```python
from build123d import *

# Parameters (mm, degrees)
F0_R     = 2.1463
F1_DEPTH = 380


with BuildPart() as f1:
    # F0 (on Front) → F1 (new body)
    with BuildSketch(Plane.XZ):
        with BuildLine():
            Line((-9.75241, 4.759444), (-12.019248, 4.759444))
            ThreePointArc((-12.019248, 4.759444), (-13.166227, 4.987592), (-14.138589, 5.637303))
            Line((-14.138589, 5.637303), (-16.393426, 7.892141))
            ThreePointArc((-16.393426, 7.892141), (-16.575125, 8.805603), (-15.800729, 9.323038))
            Line((-15.800729, 9.323038), (-13.692529, 9.323038))
            ThreePointArc((-13.692529, 9.323038), (-13.477003, 9.412312), (-13.387729, 9.627838))
            Line((-13.387729, 9.627838), (-13.387729, 10.339038))
            ThreePointArc((-13.387729, 10.339038), (-13.618353, 10.895814), (-14.175129, 11.126438))
            Line((-14.175129, 11.126438), (-18.874129, 11.126438))
            ThreePointArc((-18.874129, 11.126438), (-20.29301, 10.538718), (-20.880729, 9.119838))
            Line((-20.880729, 9.119838), (-20.880729, 4.420838))
            ThreePointArc((-20.880729, 4.420838), (-20.650105, 3.864062), (-20.093329, 3.633438))
            Line((-20.093329, 3.633438), (-19.382129, 3.633438))
            ThreePointArc((-19.382129, 3.633438), (-19.166603, 3.722712), (-19.077329, 3.938238))
            Line((-19.077329, 3.938238), (-19.077329, 6.046438))
            ThreePointArc((-19.077329, 6.046438), (-18.559895, 6.820834), (-17.646432, 6.639135))
            Line((-17.646432, 6.639135), (-15.391595, 4.384297))
            ThreePointArc((-15.391595, 4.384297), (-14.741884, 3.411936), (-14.513736, 2.264957))
            Line((-14.513736, 2.264957), (-14.513736, -0.001881))
            ThreePointArc((-14.513736, -0.001881), (-14.741884, -1.14886), (-15.391595, -2.121222))
            Line((-15.391595, -2.121222), (-17.646432, -4.376059))
            ThreePointArc((-17.646432, -4.376059), (-18.559895, -4.557758), (-19.077329, -3.783362))
            Line((-19.077329, -3.783362), (-19.077329, -1.675162))
            ThreePointArc((-19.077329, -1.675162), (-19.166603, -1.459636), (-19.382129, -1.370362))
            Line((-19.382129, -1.370362), (-20.093329, -1.370362))
            ThreePointArc((-20.093329, -1.370362), (-20.650105, -1.600986), (-20.880729, -2.157762))
            Line((-20.880729, -2.157762), (-20.880729, -6.856762))
            ThreePointArc((-20.880729, -6.856762), (-20.29301, -8.275643), (-18.874129, -8.863362))
            Line((-18.874129, -8.863362), (-14.175129, -8.863362))
            ThreePointArc((-14.175129, -8.863362), (-13.618353, -8.632738), (-13.387729, -8.075962))
            Line((-13.387729, -8.075962), (-13.387729, -7.364762))
            ThreePointArc((-13.387729, -7.364762), (-13.477003, -7.149236), (-13.692529, -7.059962))
            Line((-13.692529, -7.059962), (-15.800729, -7.059962))
            ThreePointArc((-15.800729, -7.059962), (-16.575125, -6.542528), (-16.393426, -5.629065))
            Line((-16.393426, -5.629065), (-14.138589, -3.374228))
            ThreePointArc((-14.138589, -3.374228), (-13.166227, -2.724517), (-12.019248, -2.496368))
            Line((-12.019248, -2.496368), (-9.75241, -2.496368))
            ThreePointArc((-9.75241, -2.496368), (-8.605431, -2.724517), (-7.63307, -3.374228))
            Line((-7.63307, -3.374228), (-5.378232, -5.629065))
            ThreePointArc((-5.378232, -5.629065), (-5.196534, -6.542528), (-5.970929, -7.059962))
            Line((-5.970929, -7.059962), (-8.079129, -7.059962))
            ThreePointArc((-8.079129, -7.059962), (-8.294656, -7.149236), (-8.383929, -7.364762))
            Line((-8.383929, -7.364762), (-8.383929, -8.075962))
            ThreePointArc((-8.383929, -8.075962), (-8.153305, -8.632738), (-7.596529, -8.863362))
            Line((-7.596529, -8.863362), (5.814671, -8.863362))
            ThreePointArc((5.814671, -8.863362), (6.371447, -8.632738), (6.602071, -8.075962))
            Line((6.602071, -8.075962), (6.602071, -7.364762))
            ThreePointArc((6.602071, -7.364762), (6.512797, -7.149236), (6.297271, -7.059962))
            Line((6.297271, -7.059962), (4.189071, -7.059962))
            ThreePointArc((4.189071, -7.059962), (3.414675, -6.542528), (3.596374, -5.629065))
            Line((3.596374, -5.629065), (5.851211, -3.374228))
            ThreePointArc((5.851211, -3.374228), (6.823573, -2.724517), (7.970552, -2.496368))
            Line((7.970552, -2.496368), (10.23739, -2.496368))
            ThreePointArc((10.23739, -2.496368), (11.384369, -2.724517), (12.35673, -3.374228))
            Line((12.35673, -3.374228), (14.611568, -5.629065))
            ThreePointArc((14.611568, -5.629065), (14.793266, -6.542528), (14.018871, -7.059962))
            Line((14.018871, -7.059962), (11.910671, -7.059962))
            ThreePointArc((11.910671, -7.059962), (11.695144, -7.149236), (11.605871, -7.364762))
            Line((11.605871, -7.364762), (11.605871, -8.075962))
            ThreePointArc((11.605871, -8.075962), (11.836495, -8.632738), (12.393271, -8.863362))
            Line((12.393271, -8.863362), (17.092271, -8.863362))
            ThreePointArc((17.092271, -8.863362), (18.511151, -8.275643), (19.098871, -6.856762))
            Line((19.098871, -6.856762), (19.098871, -2.157762))
            ThreePointArc((19.098871, -2.157762), (18.868247, -1.600986), (18.311471, -1.370362))
            Line((18.311471, -1.370362), (17.600271, -1.370362))
            ThreePointArc((17.600271, -1.370362), (17.384744, -1.459636), (17.295471, -1.675162))
            Line((17.295471, -1.675162), (17.295471, -3.783362))
            ThreePointArc((17.295471, -3.783362), (16.778036, -4.557758), (15.864574, -4.376059))
            Line((15.864574, -4.376059), (13.609736, -2.121222))
            ThreePointArc((13.609736, -2.121222), (12.960025, -1.14886), (12.731877, -0.001881))
            Line((12.731877, -0.001881), (12.731877, 2.264957))
            ThreePointArc((12.731877, 2.264957), (12.960025, 3.411936), (13.609736, 4.384297))
            Line((13.609736, 4.384297), (15.864574, 6.639135))
            ThreePointArc((15.864574, 6.639135), (16.778036, 6.820834), (17.295471, 6.046438))
            Line((17.295471, 6.046438), (17.295471, 3.938238))
            ThreePointArc((17.295471, 3.938238), (17.384744, 3.722712), (17.600271, 3.633438))
            Line((17.600271, 3.633438), (18.311471, 3.633438))
            ThreePointArc((18.311471, 3.633438), (18.868247, 3.864062), (19.098871, 4.420838))
            Line((19.098871, 4.420838), (19.098871, 9.119838))
            ThreePointArc((19.098871, 9.119838), (18.511151, 10.538718), (17.092271, 11.126438))
            Line((17.092271, 11.126438), (12.393271, 11.126438))
            ThreePointArc((12.393271, 11.126438), (11.836495, 10.895814), (11.605871, 10.339038))
            Line((11.605871, 10.339038), (11.605871, 9.627838))
            ThreePointArc((11.605871, 9.627838), (11.695144, 9.412312), (11.910671, 9.323038))
            Line((11.910671, 9.323038), (14.018871, 9.323038))
            ThreePointArc((14.018871, 9.323038), (14.793266, 8.805603), (14.611568, 7.892141))
            Line((14.611568, 7.892141), (12.35673, 5.637303))
            ThreePointArc((12.35673, 5.637303), (11.384369, 4.987592), (10.23739, 4.759444))
            Line((10.23739, 4.759444), (7.970552, 4.759444))
            ThreePointArc((7.970552, 4.759444), (6.823573, 4.987592), (5.851211, 5.637303))
            Line((5.851211, 5.637303), (3.596374, 7.892141))
            ThreePointArc((3.596374, 7.892141), (3.414675, 8.805603), (4.189071, 9.323038))
            Line((4.189071, 9.323038), (6.297271, 9.323038))
            ThreePointArc((6.297271, 9.323038), (6.512797, 9.412312), (6.602071, 9.627838))
            Line((6.602071, 9.627838), (6.602071, 10.339038))
            ThreePointArc((6.602071, 10.339038), (6.371447, 10.895814), (5.814671, 11.126438))
            Line((5.814671, 11.126438), (-7.596529, 11.126438))
            ThreePointArc((-7.596529, 11.126438), (-8.153305, 10.895814), (-8.383929, 10.339038))
            Line((-8.383929, 10.339038), (-8.383929, 9.627838))
            ThreePointArc((-8.383929, 9.627838), (-8.294656, 9.412312), (-8.079129, 9.323038))
            Line((-8.079129, 9.323038), (-5.970929, 9.323038))
            ThreePointArc((-5.970929, 9.323038), (-5.196534, 8.805603), (-5.378232, 7.892141))
            Line((-5.378232, 7.892141), (-7.63307, 5.637303))
            ThreePointArc((-7.63307, 5.637303), (-8.605431, 4.987592), (-9.75241, 4.759444))
        make_face()
        with Locations((-10.885829, 1.131538)):
            Circle(F0_R, mode=Mode.SUBTRACT)
        with BuildLine():
            Line((-7.257923, -0.001881), (-7.257923, 2.264957))
            ThreePointArc((-7.257923, 2.264957), (-7.029775, 3.411936), (-6.380064, 4.384297))
            Line((-6.380064, 4.384297), (-1.83051, 8.933851))
            ThreePointArc((-1.83051, 8.933851), (-0.890929, 9.323038), (0.048652, 8.933851))
            Line((0.048652, 8.933851), (4.598205, 4.384297))
            ThreePointArc((4.598205, 4.384297), (5.247916, 3.411936), (5.476064, 2.264957))
            Line((5.476064, 2.264957), (5.476064, -0.001881))
            ThreePointArc((5.476064, -0.001881), (5.247916, -1.14886), (4.598205, -2.121222))
            Line((4.598205, -2.121222), (0.048652, -6.670775))
            ThreePointArc((0.048652, -6.670775), (-0.890929, -7.059962), (-1.83051, -6.670775))
            Line((-1.83051, -6.670775), (-6.380064, -2.121222))
            ThreePointArc((-6.380064, -2.121222), (-7.029775, -1.14886), (-7.257923, -0.001881))
        make_face(mode=Mode.SUBTRACT)
        with Locations((9.103971, 1.131538)):
            Circle(F0_R, mode=Mode.SUBTRACT)
    extrude(amount=F1_DEPTH)


solid = f1.part
```
Verification items for the finished model (mm, model axes). Give positions to 0.01 mm unless a question says otherwise; leave off trailing zeros. Put each result on its own line as item: value.
Q1. Section check A-A on y = -161.5. Count the separate pieces of the cut face and the enclosed holes in it, and give its area (4 significant figures).
Result:
separate pieces: 1
enclosed holes: 3
area: 328.5 mm2
Q2. Scan lines: probe 1 along X at (y, z) = (-136, -7.25); probe 2 along X at (y, z) = (-329, 1.5); probe 3 along X at (y, z) = (-42.5, 4). Record each from-to range of solid material in increasing order. Write a range as from..to.
Result:
probe 1: -20.84..-13.41, -8.36..6.58, 11.63..19.06
probe 2: -14.51..-13, -8.77..-7.26, 5.48..6.99, 11.22..12.73
probe 3: -20.76..-19.08, -15.07..-6.7, 4.92..13.29, 17.3..18.98
Q3. Depth check by flat-ended pin: P1, Ø1.1, axis at y = -150, z = 1.5, coming from the -X side; P2, Ø8, axis at y = -243, z = 0, coming from the -X side; P3, Ø1.8, axis at x = -11, y = -110, coming from the +Z side; P4, Ø0.8, axis at x = 18, y = -255, coming from the -Z side. Enter the tip coordinate at first touch or a pass-through.
Result:
P1: x = -14.51
P2: x = -20.88
P3: z = 4.76
P4: z = -8.8
